from build123d import *

# Parameters (mm, degrees)
SKETCH1_W           = 220
SKETCH1_H           = 140
BOSS_EXTRUDE1_DEPTH = 25.4
SKETCH3_R           = 3.2
CUT_EXTRUDE1_DEPTH  = 20
CUT_EXTRUDE2_START  = -20
SKETCH2_R           = 3.2
CUT_EXTRUDE2_DEPTH  = 20


with BuildPart() as part:
    # Sketch1 → Boss-Extrude1 (new body)
    with BuildSketch(Plane(origin=(0, 0, 0), x_dir=(1, 0, 0), z_dir=(0, 1, 0))):
        Rectangle(SKETCH1_W, SKETCH1_H)
    extrude(amount=BOSS_EXTRUDE1_DEPTH)

    # Sketch3 → Cut-Extrude1 (cut)
    with BuildSketch(Plane.ZY.offset(110)):
        with Locations((-5, 12.7)):
            Circle(SKETCH3_R)
    extrude(amount=-CUT_EXTRUDE1_DEPTH, mode=Mode.SUBTRACT)

    # Sketch2 → Cut-Extrude2 (cut)
    with BuildSketch(Plane(origin=(110, 0, 0), x_dir=(0, 0, -1), z_dir=(1, 0, 0)).offset(CUT_EXTRUDE2_START)):
        with Locations(Location((5, 12.7, 0), (0, 0, 180))):
            Circle(SKETCH2_R)
    extrude(amount=CUT_EXTRUDE2_DEPTH, mode=Mode.SUBTRACT)


solid = part.part
Design review of the part built by this model. Coordinates are the model's own, in mm. A direction names the side the tool comes from. Round coordinates to 2 decimals unless told otherwise and drop trailing zeros. Loops run counter-clockwise (first coordinate to the right, second up) from the corner with the lowest first, then second, coordinate; pieces in that order, holes last. Notation, with made-up numbers: (38, 5) - (46, 5) arc R15 cw to (46, 18) - close; hole circle Ø4 at (0, 44.25). An arc over 180 degrees is marked (long way). One line per item, written item: value. Start each with the question number.
1) Insertion check: pin 1 Ø4 at (y, z) = (12.7, -5) entering from -X; pin 2 Ø1.9 at (y, z) = (13.5, -4) entering from +X. Each pin has a flat end and moves straight along its axis. Give the tip position at first contact, or say it passes through.
2) For faces 1 (the flat face through (110, 13, 1)), 2 (the flat face through (-90, 13, -5)), 3 (the cylindrical face through (99.86, 10, -3.28)), list the 3-axis set-ups (+Z, -Z, +X, -X, +Y, -Y) from which the entire face can be reached by the end or side of a thin tool; tool diameter is ignored.
3) To check wall thickness, follow L1, parallel to Y at x = 95.75, z = -5; L2, parallel to Z at x = 94.5, y = 12.7; L3, parallel to X at y = 14.25, z = -3. State the ranges of each line that lie inside material, in increasing order. Write a range as from..to.
4) Consider section A-A on z = -5. Give the boundary of the cut face in (x, y).
5) Draft analysis for pull direction Y (two halves, no side actions). For faces 4 (the cylindrical face through (-100.14, 15.4, -3.28)), 5 (the flat face through (-2, 25.4, -1)), 6 (the flat face through (90, 13, -5)), 7 (the flat face through (-2, 13, 70)), state which applies: +Y half, -Y half, draft (parallel to the pull), parting line (faces both ways), or undercut.
Reported:
1. pin 1: stops at x = -90
1. pin 2: stops at x = 90
2. face 1: +Z, -Z, +X, +Y, -Y
2. face 2: -X
2. face 3: +X
3. L1: y = 0..9.5, 15.9..25.4
3. L2: z = -70..-8.2, -1.8..70
3. L3: x = -90..90
4. outline: (-110, 0) - (110, 0) - (110, 9.5) - (90, 9.5) - (90, 15.9) - (110, 15.9) - (110, 25.4) - (-110, 25.4) - (-110, 15.9) - (-90, 15.9) - (-90, 9.5) - (-110, 9.5) - close
5. face 4: undercut
5. face 5: +Y half
5. face 6: undercut
5. face 7: draft
